Source: three-view drawing plus pictorial views. Frame: mm from the lowest corner of the part. A direction names the side the tool comes from. Give positions to 0.01 mm unless a question says otherwise; leave off trailing zeros. Order: outer loops, then holes, each group sorted by start corner. A loop starts at its lowest first (then second) coordinate and runs counter-clockwise, first axis right, second up.
1) Section A-A, the plane z = 6.75. Give the number of separate pieces and of enclosed holes in the cut face.
2) Draft query along Y for the marked faces 5, 6 and 7. Return one class per face: released by +Y, released by -Y, zero draft, split by the parting line, or undercut.
3) First-contact query: P1, Ø1.5, axis at y = 8, z = 4.5, coming from the -X side (1 decimal); P2, Ø5, axis at y = 12, z = 5.5, coming from the -X side; P3, Ø1.9, axis at y = 10.5, z = 4.5, coming from the +X side. Flat tips, straight axial feed; report the tip coordinate or a pass-through.
4) Section D-D, the plane z = 8.75. Return loops of the section in (x, y) (1 decimal).
5) Access query for the marked faces 1, 2, 3 and 4. Directions: +Z, -Z, +X, -X, +Y, -Y. A direction counts if a zero-diameter tool reaches every point of the face in a straight line with its end or side. Return the directions, or none.
6) Section C-C, the plane y = 9.75. Return loops of the section in (x, z).
7) Section B-B, the plane x = 3.6. Return loops of the section in (y, z) (1 decimal).
8) Material intervals for line 1 (Y direction, x = 3.5, z = 6.5) (1 decimal); line 2 (Z direction, x = 4, y = 9); line 3 (Y direction, x = 1, z = 2.5) (1 decimal), sorted ascending.
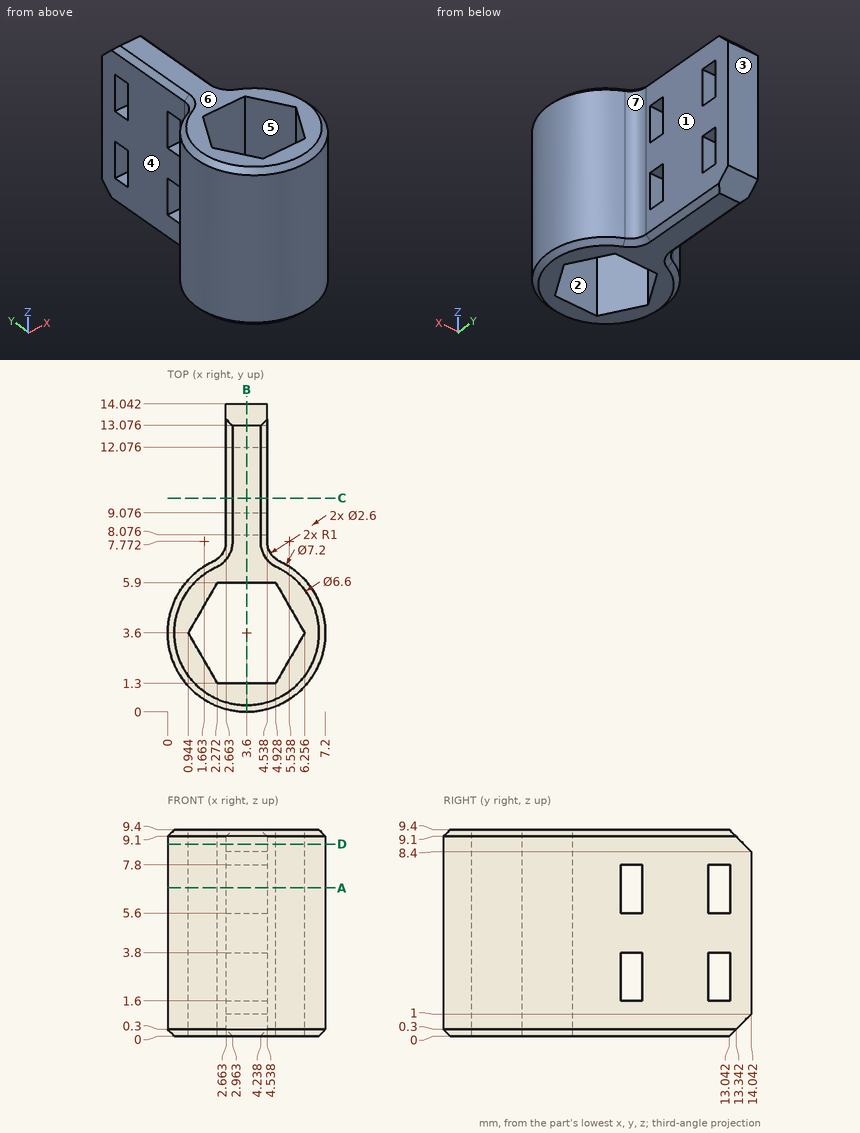
From the geometry:
1. separate pieces: 3
1. enclosed holes: 1
2. face 5: undercut
2. face 6: zero draft
2. face 7: released by +Y
3. P1: stops at x = 2.5
3. P2: stops at x = 2.66
3. P3: stops at x = 4.54
4. outline: (2.1, 6.9) arc R3.6 ccw (long way) to (5.1, 6.9) arc R1 cw to (4.5, 7.8) - (4.5, 13.7) - (2.7, 13.7) - (2.7, 7.8) arc R1 cw to start; hole (0.9, 3.6) - (2.3, 1.3) - (4.9, 1.3) - (6.3, 3.6) - (4.9, 5.9) - (2.3, 5.9) - close
5. face 1: +Z, -Z, +X, +Y
5. face 2: +Z, -Z
5. face 3: +Z, -Z, +X, -X, +Y
5. face 4: +Z, -Z, -X, +Y
6. outline: (2.66, 0.3) - (2.96, 0) - (4.24, 0) - (4.54, 0.3) - (4.54, 9.1) - (4.24, 9.4) - (2.96, 9.4) - (2.66, 9.1) - close
7. outline: (0, 0.3) - (0.3, 0) - (1.3, 0) - (1.3, 9.4) - (0.3, 9.4) - (0, 9.1) - close; (5.9, 0) - (13, 0) - (14, 1) - (14, 8.4) - (13, 9.4) - (5.9, 9.4) - close; hole (8.1, 1.6) - (9.1, 1.6) - (9.1, 3.8) - (8.1, 3.8) - close; hole (8.1, 5.6) - (9.1, 5.6) - (9.1, 7.8) - (8.1, 7.8) - close; hole (12.1, 1.6) - (13.1, 1.6) - (13.1, 3.8) - (12.1, 3.8) - close; hole (12.1, 5.6) - (13.1, 5.6) - (13.1, 7.8) - (12.1, 7.8) - close
8. line 1: y = 0 to 1.3, 5.9 to 8.1, 9.1 to 12.1, 13.1 to 14
8. line 2: z = 0 to 1.6, 3.8 to 5.6, 7.8 to 9.4
8. line 3: y = 1.1 to 3.5, 3.7 to 6.1
